Autodesk Inventor part; units mm, degrees
ref_plane "YZ Plane" through (0, 0, 0) normal (1, 0, 0) x (0, 1, 0)
ref_plane "XZ Plane" through (0, 0, 0) normal (0, 1, 0) x (-1, 0, 0)
ref_plane "XY Plane" through (0, 0, 0) normal (0, 0, 1) x (1, 0, 0)
sketch "Sketch1" plane through (0, 0, 0) normal (0, 1, 0) x (-1, 0, 0)
  circle A0 centre (0, 0) radius 1.5
  dimension "d0" = 3
extrude "Extrusion1" add sketch "Sketch1" along normal blind 12
sketch "Sketch2" plane through (0, 12, 0) normal (0, 1, 0) x (1, 0, 0)
  circle A0 centre (0, 0) radius 2
  dimension "d3" = 4
extrude "Extrusion2" add sketch "Sketch2" along normal blind 50
thread "Thread1"
fillet "Fillet1" radius 1.5 1 edges at (1.5, 0, 0)
sketch "Sketch6" plane through (0, 62, 0) normal (0, 1, 0) x (1, 0, 0)
  line L0 (4, 3) -> (-4, 3)
  line L1 (-4, 3) -> (-4, -3)
  line L2 (-4, -3) -> (4, -3)
  line L3 (4, -3) -> (4, 3)
  line L4 (4, 3) -> (-4, -3) construction
  line L5 (-4, 3) -> (4, -3) construction
  point P0 (0, 0)
  point P1 (0, 0)
  dimension "d49" = 8
  dimension "d50" = 6
  dimension "d51" = 4
  dimension "d52" = 3
  dimension "d53" = 4
  dimension "d54" = 3
extrude "Extrusion6" add sketch "Sketch6" along normal blind 3
sketch "Sketch7" plane through (0, 65, 0) normal (0, 1, 0) x (1, 0, 0)
  line L0 (-4, -3) -> (4, -3)
  line L1 (4, -3) -> (4, -1.5)
  line L2 (4, -1.5) -> (-4, -1.5)
  line L3 (-4, -1.5) -> (-4, -3)
  line L4 (4, 3) -> (-4, 3)
  line L5 (-4, 3) -> (4, 3)
  line L6 (4, 3) -> (4, 1.5)
  line L7 (4, 1.5) -> (-4, 1.5)
  line L8 (-4, 1.5) -> (-4, 3)
  point P0 (0, 0)
  point P1 (0, 0)
  dimension "d57" = 1.5
  dimension "d58" = 1.5
  dimension "d59" = 4.5
  dimension "d60" = 8
  dimension "d61" = 8
  dimension "d62" = 3
  dimension "d63" = 4
  dimension "d64" = 0
  dimension "d65" = 4
  dimension "d66" = 3
extrude "Extrusion7" add sketch "Sketch7" along normal blind 10
sketch "Sketch8" plane through (4, 62, -3) normal (0, 0, -1) x (-1, 0, 0)
  line L0 (8, 0) -> (0, 0)
  circle A0 centre (4, 10) radius 1.75
  point P0 (4, -62)
  point P1 (4, -62)
  dimension "d69" = 3.5
  dimension "d70" = 62
  dimension "d71" = 10
  dimension "d72" = 62
  dimension "d73" = 62.1289
  dimension "d74" = 72
  dimension "d75" = 0
  dimension "d76" = 62.1289
extrude "Extrusion8" cut sketch "Sketch8" against normal through all
fillet "Fillet5" radius 4 4 edges at (-4, 75, -2.25) (-4, 75, 2.25) (4, 75, -2.25) (4, 75, 2.25)
fillet "Fillet6" radius 2 1 edges at (-2, 62, 0)
properties part number "reverse gear steam chest rod valve 1"
Build history of the part. All positions in model axes, mm. A direction names the side the tool comes from. Round coordinates to 2 decimals unless told otherwise and drop trailing zeros. Order: outer loops, then holes, each group sorted by start corner. A loop starts at its lowest first (then second) coordinate and runs counter-clockwise, first axis right, second up. Notation, with made-up numbers: (21, 70) - (38, 70) arc R17 cw to (38, 77) - close; hole circle Ø10 at (34.5, -30). An arc over 180 degrees is marked (long way). Use a Markdown table: item, result.
1) Pull direction X, two halves, no side cores. Call faces 1 (the face through (0.38, 70.29, 2.24)), 2 (the face through (3.5, 62, -2.3)), 3 (the face through (0.38, 70.29, -2.26)), 4 (the face through (1.5, 6.68, -0.07)): pulls with the +X half, pulls with the -X half, needs draft (parallel to the pull), parting line crosses it, or undercut.
Recorded:
| item | result |
|---|---|
| face 1 | undercut |
| face 2 | needs draft |
| face 3 | undercut |
| face 4 | parting line crosses it |
2) Flat gauge pins, fed straight in: pin 1 Ø1.1 at (x, z) = (-3.5, 1) entering from -Y; pin 2 Ø0.7 at (x, z) = (-3.5, -1.5) entering from -Y; pin 3 Ø2.5 at (x, z) = (1, -0.5) entering from +Y; pin 4 Ø2 at (x, y) = (0, 72) entering from +Z. Where does each tip first touch, or does it go through?
Recorded:
| item | result |
|---|---|
| pin 1 | stops at y = 61.78 |
| pin 2 | stops at y = 61.93 |
| pin 3 | stops at y = 74.99 |
| pin 4 | passes through |
3) Saw through at C-C on y = 7. Write the cut outline in (x, z), and give its area (3 significant figures).
Recorded:
| item | result |
|---|---|
| outline | circle Ø3 at (0, 0) |
| area | 7.07 mm² |
4) Saw through at B-B on y = 49. Write the cut outline in (x, z).
Recorded:
| item | result |
|---|---|
| outline | circle Ø4 at (0, 0) |
5) Saw through at A-A on y = 72. Write the cut outline in (x, z).
Recorded:
| item | result |
|---|---|
| outline | (-3.87, -3) - (-1.75, -3) - (-1.75, -1.5) - (-3.87, -1.5) - close; (-3.87, 1.5) - (-1.75, 1.5) - (-1.75, 3) - (-3.87, 3) - close; (1.75, -3) - (3.87, -3) - (3.87, -1.5) - (1.75, -1.5) - close; (1.75, 1.5) - (3.87, 1.5) - (3.87, 3) - (1.75, 3) - close |
6) Tool access for faces 5 (the face through (-3.5, 62, 2.3)), 6 (the face through (0, 65, 0)), 7 (the face through (-3.6, 62, -2.4)): list every direction of +Z, -Z, +X, -X, +Y, -Y with a clear straight run to the whole face (end or side of a thin tool).
Recorded:
| item | result |
|---|---|
| face 5 | +Z, -X, -Y |
| face 6 | +X, -X, +Y |
| face 7 | -Z, -X, -Y |
7) Wall check: L1, parallel to Z at x = 0.25, y = 33; L2, parallel to X at y = 72, z = 1.85; L3, parallel to Y at x = -1, z = 2. Give the ranges that are in metal, low to high.
Recorded:
| item | result |
|---|---|
| L1 | z = -1.98 to 1.98 |
| L2 | x = -3.87 to -1.75, 1.75 to 3.87 |
| L3 | y = 60.94 to 70.56, 73.44 to 74.87 |
